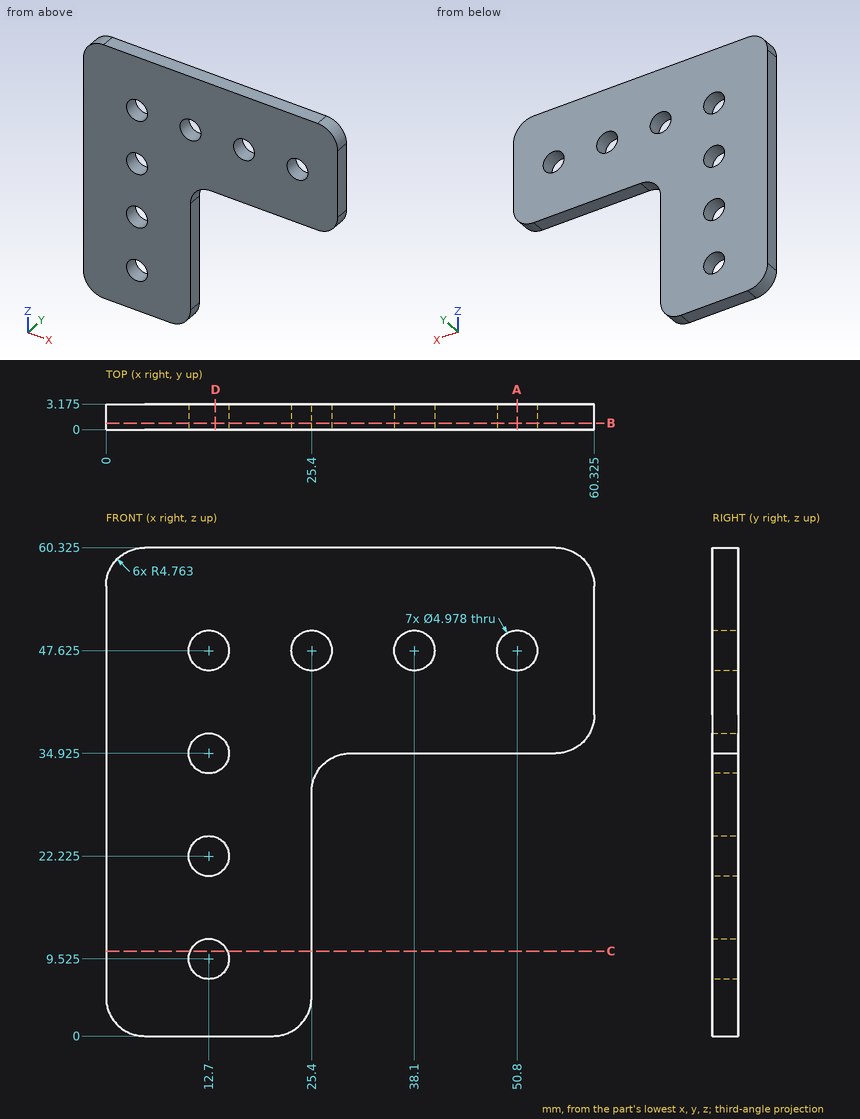
Geometry check sheet. Reference: drawing and pictorial views, mm from the part's lowest x, y, z. Give positions to 0.01 mm unless a question says otherwise; leave off trailing zeros. Order: outer loops, then holes, each group sorted by start corner. A loop starts at its lowest first (then second) coordinate and runs counter-clockwise, first axis right, second up. Notation, with made-up numbers: (84.5, -38.5) - (107.5, -38.5) arc R28 cw to (107.5, -4.5) - close; hole circle Ø9 at (48.25, 35.5). An arc over 180 degrees is marked (long way). Answer as CSV lines item,"result".
1. Section check C-C (z = 10.5). Record the boundary of the cut face in (x, y) (1 decimal).
Result sheet:
outline,"(0, 0) - (10.4, 0) - (10.4, 3.2) - (0, 3.2) - close; (15, 0) - (25.4, 0) - (25.4, 3.2) - (15, 3.2) - close"
2. Go/stop test with flat-tipped pins: P1, Ø3, axis at x = 12.7, z = 22.225, coming from the -Y side; P2, Ø1.6, axis at x = 47, y = 2, coming from the -Z side (1 decimal). Record where each tip stops, or that it passes through.
Result sheet:
P1,"through"
P2,"z = 34.9"
3. Scan lines: probe 1 along Z at (x, y) = (12.5, 2.85) (1 decimal); probe 2 along X at (y, z) = (2.85, 49.5) (1 decimal); probe 3 along Z at (x, y) = (38, 2.9) (1 decimal). Record each from-to range of solid material in increasing order. Write a range as from..to.
Result sheet:
probe 1,"0..7, 12..19.7, 24.7..32.4, 37.4..45.1, 50.1..60.3"
probe 2,"0..11.1, 14.3..23.8, 27..36.5, 39.7..49.2, 52.4..60.3"
probe 3,"34.9..45.1, 50.1..60.3"
4. Section check B-B (y = 0.8). Record the boundary of the cut face in (x, z) (1 decimal), then the cut area to 3 significant figures.
Result sheet:
outline,"(0, 4.8) arc R4.8 ccw to (4.8, 0) - (20.6, 0) arc R4.8 ccw to (25.4, 4.8) - (25.4, 30.2) arc R4.8 cw to (30.2, 34.9) - (55.6, 34.9) arc R4.8 ccw to (60.3, 39.7) - (60.3, 55.6) arc R4.8 ccw to (55.6, 60.3) - (4.8, 60.3) arc R4.8 ccw to (0, 55.6) - close; hole circle Ø5 at (12.7, 9.5); hole circle Ø5 at (12.7, 22.2); hole circle Ø5 at (12.7, 34.9); hole circle Ø5 at (12.7, 47.6); hole circle Ø5 at (25.4, 47.6); hole circle Ø5 at (38.1, 47.6); hole circle Ø5 at (50.8, 47.6)"
area,"2,260 mm²"
5. Section check D-D (x = 13.5). Record the boundary of the cut face in (y, z) (1 decimal), then the cut area to 3 significant figures.
Result sheet:
outline,"(0, 0) - (3.2, 0) - (3.2, 7.2) - (0, 7.2) - close; (0, 11.9) - (3.2, 11.9) - (3.2, 19.9) - (0, 19.9) - close; (0, 24.6) - (3.2, 24.6) - (3.2, 32.6) - (0, 32.6) - close; (0, 37.3) - (3.2, 37.3) - (3.2, 45.3) - (0, 45.3) - close; (0, 50) - (3.2, 50) - (3.2, 60.3) - (0, 60.3) - close"
area,"132 mm²"
6. Section check A-A (x = 50.8). Record the boundary of the cut face in (y, z) (1 decimal).
Result sheet:
outline,"(0, 34.9) - (3.2, 34.9) - (3.2, 45.1) - (0, 45.1) - close; (0, 50.1) - (3.2, 50.1) - (3.2, 60.3) - (0, 60.3) - close"
